Build history of the part. All positions in model axes, mm. Coordinates: 2 decimals unless noted, no trailing zeros. Loops run counter-clockwise (first coordinate to the right, second up) from the corner with the lowest first, then second, coordinate; pieces in that order, holes last.
Item 1: Cut at D-D (y = 14.1). List the corners of the cut face in (x, z), and give its area (3 significant figures).
Item 2: Drill centre lines: line 1 along Y through (x, z) = (1.4, 0.2); line 2 along X through (y, z) = (12, 0.1); line 3 along Y through (x, z) = (1.2, 0.1). Where is each one in solid material? Low to high.
Item 3: Cut at C-C (x = 1.4). List the corners of the cut face in (y, z), and give its area (3 significant figures).
Item 4: Cut at A-A (y = 3.75). List the corners of the cut face in (x, z), and give its area (3 significant figures).
Item 5: Cut at B-B (x = 2). List the corners of the cut face in (y, z), and give its area (3 significant figures).
from build123d import *

# Parameters (mm, degrees)
SKETCH1_W           = 2
SKETCH1_H           = 4.09895497
SKETCH1_H_2         = 4.100689225
BOSS_EXTRUDE1_DEPTH = 0.3
SKETCH2_R           = 0.25
CUT_EXTRUDE2_DEPTH  = 0.3
FILLET10_R          = 0.15


with BuildPart() as part:
    # Sketch1 → Boss-Extrude1 (new body)
    with BuildSketch(Plane.XY):
        with BuildLine():
            Line((0, 0), (0, 4.600689225))
            Line((0, 4.600689225), (0.4, 5))
            Line((0.4, 5), (0.4, 8.5))
            Line((0.4, 8.5), (0, 8.90104503))
            Line((0, 8.90104503), (0, 13.5))
            ThreePointArc((0, 13.5), (1.4, 14.9), (2.8, 13.5))
            Line((2.8, 13.5), (2.8, 8.900318658))
            Line((2.8, 8.900318658), (2.4, 8.5))
            Line((2.4, 8.5), (2.4, 5))
            Line((2.4, 5), (2.8, 4.60077765))
            Line((2.8, 4.60077765), (2.8, 0))
            ThreePointArc((2.8, 0), (1.4, -1.4), (0, 0))
        make_face()
        with Locations((1.4, 11.450522515)):
            Rectangle(SKETCH1_W, SKETCH1_H, mode=Mode.SUBTRACT)
        with Locations((1.4, 2.050344612)):
            Rectangle(SKETCH1_W, SKETCH1_H_2, mode=Mode.SUBTRACT)
    extrude(amount=BOSS_EXTRUDE1_DEPTH)

    # Sketch2 → Cut-Extrude2 (cut)
    with BuildSketch(Plane.XY.offset(0.3)):
        with Locations((1.4, 8.199310775)):
            Circle(SKETCH2_R)
        with Locations((2, 14.1)):
            Circle(SKETCH2_R)
        with Locations((1.4, 5.300689225)):
            Circle(SKETCH2_R)
        with Locations((0.8, 14.1)):
            Circle(SKETCH2_R)
        with BuildLine():
            ThreePointArc((1.807854557, -0.440062109), (2.176776695, -0.776776695), (1.840062109, -0.407854557))
            ThreePointArc((1.840062109, -0.407854557), (1.824264069, -0.424264069), (1.807854557, -0.440062109))
        make_face()
        with BuildLine():
            ThreePointArc((0.992145443, -0.440062109), (0.975735931, -0.424264069), (0.959937891, -0.407854557))
            ThreePointArc((0.959937891, -0.407854557), (0.623223305, -0.776776695), (0.992145443, -0.440062109))
        make_face()
        with Locations((0.8, 4.700689225)):
            Circle(SKETCH2_R)
        with Locations((2, 4.700689225)):
            Circle(SKETCH2_R)
        with Locations((2, 8.799310775)):
            Circle(SKETCH2_R)
        with Locations((0.8, 8.799310775)):
            Circle(SKETCH2_R)
    extrude(amount=-CUT_EXTRUDE2_DEPTH, mode=Mode.SUBTRACT)

    # Fillet10
    fillet10_edges = [part.edges().sort_by_distance(p)[0] for p in [
        (0, 4.600689225, 0.15),
        (0.4, 5, 0.15),
        (0.4, 8.5, 0.15),
        (0, 8.90104503, 0.15),
        (2.8, 8.900318658, 0.15),
        (2.4, 8.5, 0.15),
        (2.4, 5, 0.15),
        (2.8, 4.60077765, 0.15),
    ]]
    fillet(fillet10_edges, radius=FILLET10_R)


solid = part.part
Filled sheet:
1. outline: (0.14, 0) - (0.55, 0) - (0.55, 0.3) - (0.14, 0.3) - close; (1.05, 0) - (1.75, 0) - (1.75, 0.3) - (1.05, 0.3) - close; (2.25, 0) - (2.66, 0) - (2.66, 0.3) - (2.25, 0.3) - close
1. area: 0.459 mm2
2. line 1: y = -1.4 to 0, 4.1 to 5.05, 5.55 to 7.95, 8.45 to 9.4, 13.5 to 14.9
2. line 2: x = 0 to 0.4, 2.4 to 2.8
2. line 3: y = -1.39 to 0, 4.1 to 5.15, 5.45 to 8.05, 8.35 to 9.4, 13.5 to 14.89
3. outline: (-1.4, 0) - (0, 0) - (0, 0.3) - (-1.4, 0.3) - close; (4.1, 0) - (5.05, 0) - (5.05, 0.3) - (4.1, 0.3) - close; (5.55, 0) - (7.95, 0) - (7.95, 0.3) - (5.55, 0.3) - close; (8.45, 0) - (9.4, 0) - (9.4, 0.3) - (8.45, 0.3) - close; (13.5, 0) - (14.9, 0) - (14.9, 0.3) - (13.5, 0.3) - close
3. area: 2.13 mm2
4. outline: (0, 0) - (0.4, 0) - (0.4, 0.3) - (0, 0.3) - close; (2.4, 0) - (2.8, 0) - (2.8, 0.3) - (2.4, 0.3) - close
4. area: 0.240 mm2
5. outline: (-1.26, 0) - (-0.85, 0) - (-0.85, 0.3) - (-1.26, 0.3) - close; (-0.35, 0) - (0, 0) - (0, 0.3) - (-0.35, 0.3) - close; (4.1, 0) - (4.45, 0) - (4.45, 0.3) - (4.1, 0.3) - close; (4.95, 0) - (8.55, 0) - (8.55, 0.3) - (4.95, 0.3) - close; (9.05, 0) - (9.4, 0) - (9.4, 0.3) - (9.05, 0.3) - close; (13.5, 0) - (13.85, 0) - (13.85, 0.3) - (13.5, 0.3) - close; (14.35, 0) - (14.76, 0) - (14.76, 0.3) - (14.35, 0.3) - close
5. area: 1.75 mm2
